Can you work these out from the model? Positions are in its coordinate system, mm. A direction names the side the tool comes from. Round coordinates to 2 decimals unless told otherwise and drop trailing zeros. Loops run counter-clockwise (first coordinate to the right, second up) from the corner with the lowest first, then second, coordinate; pieces in that order, holes last.
from build123d import *

# Parameters (mm, degrees)
BOSS_EXTRUDE1_DEPTH = 63
SKETCH4_W           = 10.621571424
SKETCH4_H           = 15.75
SKETCH4_R           = 3.1
CUT_EXTRUDE5_DEPTH  = 63


with BuildPart() as part:
    # Sketch3 → Boss-Extrude1 (new body)
    with BuildSketch(Plane.XY):
        with BuildLine():
            Line((0, 0), (31, 0))
            ThreePointArc((31, 0), (33.641651825, 1.402050733), (34.697848077, 4.2))
            ThreePointArc((34.697848077, 4.2), (30.061245163, 7.776705153), (27.778786239, 2.383998263))
            Line((27.778786239, 2.383998263), (29.520996138, 3.366192068))
            ThreePointArc((29.520996138, 3.366192068), (30.568975506, 5.842225922), (32.697848077, 4.2))
            ThreePointArc((32.697848077, 4.2), (32.224028116, 2.810513756), (31, 2))
            Line((31, 2), (28.027781906, 2))
            Line((28.027781906, 2), (0, 2))
            Line((0, 2), (0, 0))
        make_face()
    extrude(amount=-BOSS_EXTRUDE1_DEPTH)

    # Sketch4 → Cut-Extrude5 (cut)
    with BuildSketch(Plane(origin=(0, 12, 0), x_dir=(1, 0, 0), z_dir=(0, 1, 0))):
        with Locations((32.491992857, 39.375)):
            Rectangle(SKETCH4_W, SKETCH4_H)
        with Locations((32.491992857, 7.875)):
            Rectangle(SKETCH4_W, SKETCH4_H)
        with Locations(Location((10, 13, 0), (0, 0, 270))):
            Circle(SKETCH4_R)
        with Locations(Location((10, 50, 0), (0, 0, 270))):
            Circle(SKETCH4_R)
    extrude(amount=-CUT_EXTRUDE5_DEPTH, mode=Mode.SUBTRACT)


solid = part.part
(1) If we section it at B-B, the plane z = -29.5: List the corners of the cut face in (x, y) for me.
Worked answers:
outline: (0, 0) - (31, 0) arc R4.23 ccw to (34.7, 4.2) arc R3.7 ccw (long way) to (27.78, 2.38) - (29.52, 3.37) arc R1.7 cw (long way) to (32.7, 4.2) arc R2.27 cw to (31, 2) - (0, 2) - close
(2) If we mould it in two halves opening along Y, with no side actions, what happens to faces 6 (the cylindrical face through (32.24, 2.83, -55.01)), 7 (the cylindrical face through (10.1, 1, -16.1)), 8 (the flat face through (15, 0, -31))? For each: released by +Y, released by -Y, zero draft, split by the parting line, or undercut.
Worked answers:
face 6: undercut
face 7: zero draft
face 8: released by -Y
(3) If we section it at D-D, the plane z = -49: List the corners of the cut face in (x, y) for me.
Worked answers:
outline: (0, 0) - (7.07, 0) - (7.07, 2) - (0, 2) - close; (12.93, 0) - (31, 0) arc R4.23 ccw to (34.7, 4.2) arc R3.7 ccw (long way) to (27.78, 2.38) - (29.52, 3.37) arc R1.7 cw (long way) to (32.7, 4.2) arc R2.27 cw to (31, 2) - (12.93, 2) - close
(4) Will these pins go through, and if not, where does the flat tip stop? P1, Ø8, axis at x = 10, z = -50, coming from the -Y side; P2, Ø4, axis at x = 31, y = 4.2, coming from the +Z side; P3, Ø1.5, axis at x = 18.5, z = -6.5, coming from the +Y side; P4, Ø1, axis at y = 1.5, z = -42, coming from the +X side.
Worked answers:
P1: stops at y = 0
P2: stops at z = -15.75
P3: stops at y = 2
P4: stops at x = 27.18
(5) If I drill on line 1 (X direction, y = 1.35, z = -13); line 2 (Z direction, x = 33, y = 4.5); line 3 (Y direction, x = 2, z = -20), over which ranges is the centre line in solid material (lowest first)?
Worked answers:
line 1: x = 0 to 6.9, 13.1 to 27.18
line 2: z = -63 to -47.25, -31.5 to -15.75
line 3: y = 0 to 2
(6) If we section it at A-A, the plane z = -13: List the corners of the cut face in (x, y) for me.
Worked answers:
outline: (0, 0) - (6.9, 0) - (6.9, 2) - (0, 2) - close; (13.1, 0) - (27.18, 0) - (27.18, 2) - (13.1, 2) - close
(7) For faces 1 (the flat face through (27.181, 1, -39)), 2 (the cylindrical face through (33.613, 1.37, -55.015)), 3 (the flat face through (29, 4, -15.75)), 4 (the flat face through (28.64, 2.87, -55.01)), 5 (the flat face through (19.8, 1.6, -63)), which set-ups out of +Z, -Z, +X, -X, +Y, -Y let a thin tool reach every point of the face, with its end or its side?
Worked answers:
face 1: +X, +Y, -Y
face 2: +Z, -Z, +X, -Y
face 3: +Z, +X, +Y, -Y
face 4: +Z, -Z
face 5: -Z, +X, -X, +Y, -Y
(8) If we section it at C-C, the plane x = 14: List the corners of the cut face in (y, z) for me, then the cut area to 3 significant figures.
Worked answers:
outline: (0, -63) - (2, -63) - (2, 0) - (0, 0) - close
area: 126 mm2
